Design review of the part built by this model. Coordinates are the model's own, in mm. Face numbers are marked on the shaded views. A direction names the side the tool comes from. Round coordinates to 2 decimals unless told otherwise and drop trailing zeros. Write each loop counter-clockwise with the first axis right and the second up, starting at its lowest first coordinate (ties: lowest second). Pieces come first, ordered by that corner, then holes. Notation, with made-up numbers: (62.5, 86.5) -> (90.5, 86.5) arc R34 cw to (90.5, 120.5) -> close; hole circle Ø6 at (24, -39). An arc over 180 degrees is marked (long way). Write item = value, one per line. Start each with the question number.
Item 1: Add section C-C, the plane x = -39.5. State the section outline as (y, z) points, then the cut area to 3 significant figures.
Item 2: Add section D-D, the plane y = 11. State the section outline as (x, z) points.
Item 3: Mouldability with a two-part tool opening along Z and no side actions: class the marked faces 1, 2 and 3 as released by +Z, released by -Z, zero draft, split by the parting line, or undercut.
Item 4: Machinability: for the marked faces 4 and 5, which of the approach directions +Z, -Z, +X, -X, +Y, -Y give a long, thin tool a straight path to every point of the face, cutting with its end or side? Answer none if there is none.
Item 5: For pin 1 Ø10 at (x, y) = (-38.42, 82.55) entering from +Z; pin 2 Ø15 at (y, z) = (-23.5, 14) entering from -X; pin 3 Ø3 at (y, z) = (-84, 21) entering from +X; pin 4 Ø7 at (y, z) = (-10, 2) entering from +X, all flat-tipped, find the tip position at first contact; note any pin that passes through.
Item 6: Add section A-A, the plane y = -82.55. State the section outline as (x, z) points.
Item 7: Add section B-B, the plane z = 21. State the section outline as (x, y) points.
Item 8: To check wall thickness, follow L1, parallel to X at y = -82, z = 2; L2, parallel to Z at x = 33.5, y = -51.5; L3, parallel to X at y = 70, z = 19. State the ranges of each line that lie inside material, in increasing order.
from build123d import *

# Parameters (mm, degrees)
SKETCH2_R           = 6.35
BOSS_EXTRUDE1_DEPTH = 6.35
BOSS_EXTRUDE7_DEPTH = 203.2
BOSS_EXTRUDE8_START = 50.8
SKETCH4_R           = 25.4
BOSS_EXTRUDE8_DEPTH = 50.8
SKETCH5_R           = 21.02866
CUT_EXTRUDE2_DEPTH  = 265.465112255
FILLET1_R           = 6.35


with BuildPart() as part:
    # Sketch2 → Boss-Extrude1 (new body)
    with BuildSketch(Plane.XY):
        Polygon((-53.34, -101.6), (53.34, -101.6), (53.34, -63.5), (31.75, -26.105023065), (31.75, 26.105023065), (53.34, 63.5), (53.34, 101.6), (-53.34, 101.6), (-53.34, 63.5), (-31.75, 26.105023065), (-31.75, -26.105023065), (-53.34, -63.5), align=None)
        with Locations((-38.4175, 82.55)):
            Circle(SKETCH2_R, mode=Mode.SUBTRACT)
        with Locations(Location((-38.4175, -82.55, 0), (0, 0, 180))):
            Circle(SKETCH2_R, mode=Mode.SUBTRACT)
        with Locations((38.4175, -82.55)):
            Circle(SKETCH2_R, mode=Mode.SUBTRACT)
        with Locations(Location((38.4175, 82.55, 0), (0, 0, 180))):
            Circle(SKETCH2_R, mode=Mode.SUBTRACT)
    extrude(amount=BOSS_EXTRUDE1_DEPTH)

    # Sketch3 → Boss-Extrude7 (add)
    with BuildSketch(Plane.XZ.offset(101.6)):
        with BuildLine():
            Line((-25.4, 25.4), (-25.4, 6.35))
            Line((-25.4, 6.35), (-16.800520825, 6.35))
            ThreePointArc((-16.800520825, 6.35), (0, 0), (16.800520825, 6.35))
            Line((16.800520825, 6.35), (25.4, 6.35))
            Line((25.4, 6.35), (25.4, 25.4))
            ThreePointArc((25.4, 25.4), (0, 50.8), (-25.4, 25.4))
        make_face()
    extrude(amount=-BOSS_EXTRUDE7_DEPTH)

    # Sketch4 → Boss-Extrude8 (add)
    with BuildSketch(Plane.XZ.offset(101.6).offset(BOSS_EXTRUDE8_START)):
        with Locations(Location((0, 25.4, 0), (0, 0, 270))):
            Circle(SKETCH4_R)
    extrude(amount=-BOSS_EXTRUDE8_DEPTH)

    # Sketch5 → Cut-Extrude2 (cut, through all)
    with BuildSketch(Plane.XZ.offset(152.4)):
        with Locations(Location((0, 25.4, 0), (0, 0, 270))):
            Circle(SKETCH5_R)
    extrude(amount=-CUT_EXTRUDE2_DEPTH, mode=Mode.SUBTRACT)

    # Fillet1
    fillet1_edges = [part.edges().sort_by_distance(p)[0] for p in [
        (53.34, 63.5, 3.175),
        (31.75, 26.105023065, 3.175),
        (31.75, -26.105023065, 3.175),
        (53.34, -63.5, 3.175),
        (53.34, -101.6, 3.175),
        (-53.34, -101.6, 3.175),
        (-53.34, -63.5, 3.175),
        (-31.75, -26.105023065, 3.175),
        (-31.75, 26.105023065, 3.175),
        (-53.34, 63.5, 3.175),
        (-53.34, 101.6, 3.175),
        (53.34, 101.6, 3.175),
    ]]
    fillet(fillet1_edges, radius=FILLET1_R)


solid = part.part
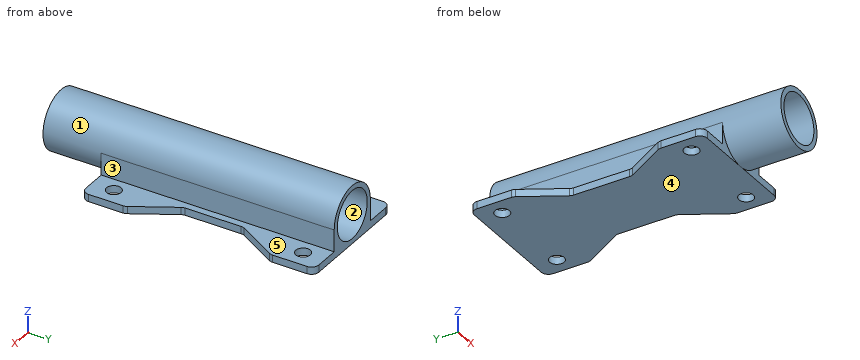
Result set:
q1.outline = (-101.6, 0) -> (-88.81, 0) -> (-88.81, 6.35) -> (-101.6, 6.35) -> close; (-76.29, 0) -> (-39.53, 0) -> (-39.53, 6.35) -> (-76.29, 6.35) -> close; (39.53, 0) -> (76.29, 0) -> (76.29, 6.35) -> (39.53, 6.35) -> close; (88.81, 0) -> (101.6, 0) -> (101.6, 6.35) -> (88.81, 6.35) -> close
q1.area = 629 mm²
q2.outline = (-31.75, 0) -> (31.75, 0) -> (31.75, 6.35) -> (25.4, 6.35) -> (25.4, 25.4) arc R25.4 ccw to (-25.4, 25.4) -> (-25.4, 6.35) -> (-31.75, 6.35) -> close; hole circle Ø42.06 at (0, 25.4)
q3.face_1 = split by the parting line
q3.face_2 = undercut
q3.face_3 = zero draft
q4.face_4 = -Z, +X, -X, +Y, -Y
q4.face_5 = +Z, +X, +Y, -Y
q5.pin_1 = through
q5.pin_2 = -25.4
q5.pin_3 = 25.4
q5.pin_4 = 31.75
q6.outline = (-53.34, 0) -> (-44.77, 0) -> (-44.77, 6.35) -> (-53.34, 6.35) -> close; (-32.07, 0) -> (32.07, 0) -> (32.07, 6.35) -> (25.4, 6.35) -> (25.4, 25.4) arc R25.4 ccw to (-25.4, 25.4) -> (-25.4, 6.35) -> (-32.07, 6.35) -> close; (44.77, 0) -> (53.34, 0) -> (53.34, 6.35) -> (44.77, 6.35) -> close; hole circle Ø42.06 at (0, 25.4)
q7.outline = (-25.4, -101.6) -> (-25.02, -101.6) -> (-25.02, -152.4) -> (-20.56, -152.4) -> (-20.56, 101.6) -> (-25.4, 101.6) -> close; (20.56, -152.4) -> (25.02, -152.4) -> (25.02, -101.6) -> (25.4, -101.6) -> (25.4, 101.6) -> (20.56, 101.6) -> close
q8.L1 = -53.34 to -44.74, -32.09 to 32.09, 44.74 to 53.34
q8.L2 = 0 to 6.35
q8.L3 = -25.4 to -20.03, 20.03 to 25.4
